Check sheet for the drawn part. Datum: minimum x, y, z corner. Units: mm. Give positions to 0.01 mm unless a question says otherwise; leave off trailing zeros. Order: outer loops, then holes, each group sorted by start corner. A loop starts at its lowest first (then second) coordinate and runs counter-clockwise, first axis right, second up.
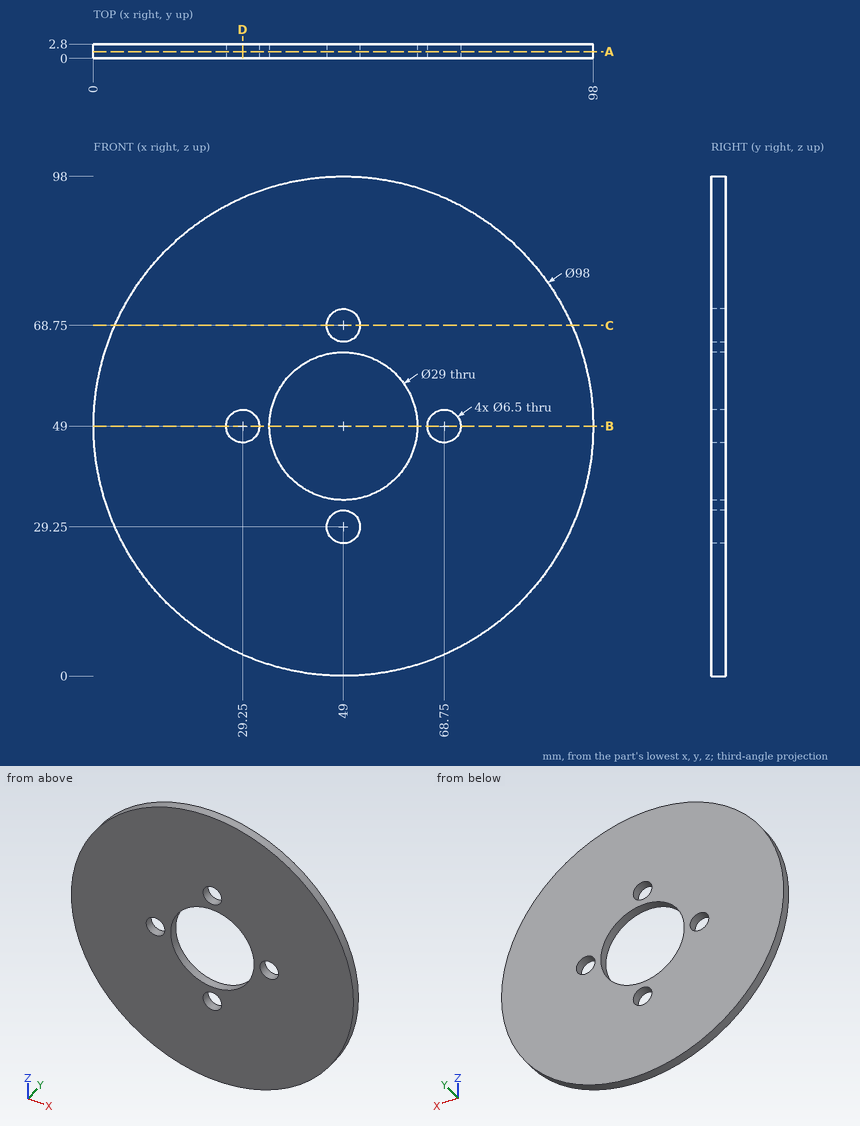
Q1. Sectioned sample at A-A, the plane y = 1.3. Record the cut outline in (x, z).
Q2. Go/stop test with a flat-tipped pin: P1, Ø1.5, axis at x = 72.5, y = 2, coming from the -Z side. Record where the tip stops, or that it passes through.
Q3. Sectioned sample at B-B, the plane z = 49. Record the cut outline in (x, y), plus the area to 3 significant figures.
Q4. Sectioned sample at D-D, the plane x = 29.25. Record the cut outline in (y, z).
Q5. Sectioned sample at C-C, the plane z = 68.75. Record the cut outline in (x, y).
Q6. Material ranges on line 1 (X direction, y = 1.2, z = 49); line 2 (X direction, y = 1.8, z = 52.5), recorded low to high.
Filled in:
1. outline: circle Ø98 at (49, 49); hole circle Ø6.5 at (29.25, 49); hole circle Ø29 at (49, 49); hole circle Ø6.5 at (49, 29.25); hole circle Ø6.5 at (49, 68.75); hole circle Ø6.5 at (68.75, 49)
2. P1: stops at z = 5.6
3. outline: (0, 0) - (26, 0) - (26, 2.8) - (0, 2.8) - close; (32.5, 0) - (34.5, 0) - (34.5, 2.8) - (32.5, 2.8) - close; (63.5, 0) - (65.5, 0) - (65.5, 2.8) - (63.5, 2.8) - close; (72, 0) - (98, 0) - (98, 2.8) - (72, 2.8) - close
3. area: 157 mm2
4. outline: (0, 4.16) - (2.8, 4.16) - (2.8, 45.75) - (0, 45.75) - close; (0, 52.25) - (2.8, 52.25) - (2.8, 93.84) - (0, 93.84) - close
5. outline: (4.16, 0) - (45.75, 0) - (45.75, 2.8) - (4.16, 2.8) - close; (52.25, 0) - (93.84, 0) - (93.84, 2.8) - (52.25, 2.8) - close
6. line 1: x = 0 to 26, 32.5 to 34.5, 63.5 to 65.5, 72 to 98
6. line 2: x = 0.13 to 34.93, 63.07 to 97.87
